Verification items for the finished model (mm, model axes). A direction names the side the tool comes from. Give positions to 0.01 mm unless a question says otherwise; leave off trailing zeros. Order: outer loops, then holes, each group sorted by start corner. A loop starts at its lowest first (then second) coordinate and runs counter-clockwise, first axis right, second up.
(1) Mould release check, pull along Z, two halves, no side actions. Record for faces 1 (the face through (5.07, 66.065, -59.466)), 2 (the face through (4.93, 26.618, -61.103)), 3 (the face through (5.07, 64.771, -156.978)), 4 (the face through (10, 56, -93)): pulls with the +Z half, pulls with the -Z half, needs draft (parallel to the pull), parting line crosses it, or undercut.
(2) Sectioned sample at A-A on z = -160. Record the cut outline in (x, y), plus the area to 3 significant figures.
(3) Scan lines: L1, parallel to Y at x = 17, z = -2.75; L2, parallel to X at y = 85.5, z = -88; L3, parallel to Z at x = -11, y = 35.5. Record each from-to range of solid material in increasing order.
(4) Sectioned sample at D-D on z = -130. Record the cut outline in (x, y).
(5) Sectioned sample at B-B on y = 62. Record the cut outline in (x, z).
(6) Sectioned sample at C-C on y = 29.5. Record the cut outline in (x, z), plus the area to 3 significant figures.
(7) Access from +Z, -Z, +X, -X, +Y, -Y to the whole of each face (thin tool, end or side, straight path). Record for faces 5 (the face through (0, 56, -93)), 6 (the face through (19, 25, -10)), 7 (the face through (5, 50, -6)), 8 (the face through (5, 52.5, -140)).
(8) Gauge pin test, flat ends, axial feed: pin 1 (3 mm diameter, centred on y = 9.5, z = -30, fed in from +X); pin 2 (10.5 mm diameter, centred on y = 62, z = -60, fed in from -X); pin 3 (4.5 mm diameter, centred on x = 12, z = -5.5, fed in from +Y); pin 4 (3 mm diameter, centred on x = -0.5, y = 64, fed in from -Z). Record the tip position at first contact, or that the pin passes through.
```python
from build123d import *

# Parameters (mm, degrees)
SALIENTE_EXTRUIR1_DEPTH = 10
SALIENTE_EXTRUIR2_DEPTH = 10
CROQUIS3_R              = 1.55
CORTAR_EXTRUIR1_DEPTH   = 10
CROQUIS4_R              = 4.1
CORTAR_EXTRUIR2_DEPTH   = 10


with BuildPart() as part:
    # Croquis1 → Saliente-Extruir1 (new body)
    with BuildSketch(Plane(origin=(0, 0, 0), x_dir=(0, 0, -1), z_dir=(1, 0, 0))):
        Polygon((0, 0), (0, 50), (15, 50), (84.282032303, 90), (173.002060716, 90), (173.002060716, 52.5), (105.932667397, 52.5), (15, 0), align=None)
    extrude(amount=SALIENTE_EXTRUIR1_DEPTH)

    # Croquis2 → Saliente-Extruir2 (add)
    with BuildSketch(Plane.XY):
        Polygon((0, 50), (-15, 50), (-15, 0), (25, 0), (25, 50), align=None)
    extrude(amount=-SALIENTE_EXTRUIR2_DEPTH)

    # Croquis3 → Cortar-Extruir1 (cut)
    with BuildSketch(Plane.XY):
        with Locations((-7, 25)):
            Circle(CROQUIS3_R)
        with Locations((17, 25)):
            Circle(CROQUIS3_R)
    extrude(amount=-CORTAR_EXTRUIR1_DEPTH, mode=Mode.SUBTRACT)

    # Croquis4 → Cortar-Extruir2 (cut)
    with BuildSketch(Plane(origin=(10, 0, 0), x_dir=(0, 0, -1), z_dir=(1, 0, 0))):
        with Locations((60, 62)):
            Circle(CROQUIS4_R)
        with Locations((160, 62)):
            Circle(CROQUIS4_R)
    extrude(amount=-CORTAR_EXTRUIR2_DEPTH, mode=Mode.SUBTRACT)


solid = part.part
```
Ans:
1. face 1: undercut
1. face 2: pulls with the -Z half
1. face 3: undercut
1. face 4: needs draft
2. outline: (0, 52.5) - (10, 52.5) - (10, 57.9) - (0, 57.9) - close; (0, 66.1) - (10, 66.1) - (10, 90) - (0, 90) - close
2. area: 293 mm2
3. L1: y = 0 to 23.45, 26.55 to 50
3. L2: x = 0 to 10
3. L3: z = -10 to 0
4. outline: (0, 52.5) - (10, 52.5) - (10, 90) - (0, 90) - close
5. outline: (0, -173) - (10, -173) - (10, -164.1) - (0, -164.1) - close; (0, -155.9) - (10, -155.9) - (10, -64.1) - (0, -64.1) - close; (0, -55.9) - (10, -55.9) - (10, -35.78) - (0, -35.78) - close
6. outline: (-15, -10) - (0, -10) - (0, -66.1) - (10, -66.1) - (10, -10) - (25, -10) - (25, 0) - (-15, 0) - close
6. area: 961 mm2
7. face 5: -Z, -X, +Y, -Y
7. face 6: -Z, +X, +Y, -Y
7. face 7: +Z, +X, -X, +Y
7. face 8: -Z, +X, -X, -Y
8. pin 1: stops at x = 10
8. pin 2: stops at x = 0
8. pin 3: stops at y = 50
8. pin 4: stops at z = -173
